Design review of the part built by this model. Coordinates are the model's own, in mm. A direction names the side the tool comes from. Give positions to 0.01 mm unless a question says otherwise; leave off trailing zeros. Write each loop counter-clockwise with the first axis right and the second up, starting at its lowest first coordinate (ties: lowest second). Pieces come first, ordered by that corner, then holes. Notation, with made-up numbers: M 70.25,52 L 87.25,52 A24 cw 87.25,63 Z; hole C -10.75,12 d4. An arc over 180 degrees is marked long. Answer in a Markdown table with one row per item.
Autodesk Inventor part; units mm, degrees
ref_plane "YZ Plane" through (0, 0, 0) normal (1, 0, 0) x (0, 1, 0)
ref_plane "XZ Plane" through (0, 0, 0) normal (0, 1, 0) x (-1, 0, 0)
ref_plane "XY Plane" through (0, 0, 0) normal (0, 0, 1) x (1, 0, 0)
sketch "Sketch1" plane through (0, 0, 0) normal (0, 0, 1) x (1, 0, 0)
  arc A0 (-25, 0) -> (25, 0) centre (0, 0) ccw
  circle A1 centre (0, 0) radius 2.5
  circle A2 centre (0, 15) radius 2.5
  line L0 (-25, 0) -> (-6, 0)
  line L1 (-6, 0) -> (-6, 15)
  arc A3 (6, 15) -> (-6, 15) centre (0, 15) ccw
  line L2 (6, 15) -> (6, 0)
  line L3 (6, 0) -> (25, 0)
  point P0 (0, 21)
  dimension "d0" = 50
  dimension "d1" = 5
  dimension "d2" = 15
  dimension "d4" = 12
extrude "Extrusion1" add sketch "Sketch1" along normal mid plane 8
hole "Hole1" at (0, 21, 0) direction (0, -1, 0) diameter 2.459 end up to surface
chamfer "Chamfer1" distance 0.5 angle 45 4 edges at (-2.5, 15, 4) (-2.5, 0, 4) (-2.5, 0, -4) (-2.5, 15, -4)
properties part number "Counterweight"
1) To check wall thickness, follow probe 1 along Y at (x, z) = (-1, 2.5); probe 2 along Z at (x, y) = (0, 19.2); probe 3 along X at (y, z) = (13, -1.25). State the ranges of each line that lie inside material, in increasing order. Write a range as [from, to].
Geometry says:
| item | result |
|---|---|
| probe 1 | [-24.98, -2.29], [2.29, 12.71], [17.29, 20.92] |
| probe 2 | [-4, -1.23], [1.23, 4] |
| probe 3 | [-6, -1.5], [1.5, 6] |
2) The part is to be moulded in two halves that separate along X. For faces 1 (the face through (6, 8, 0)), 2 (the face through (0.55, -24.994, -0.056)), 3 (the face through (15, 0, 0)), 4 (the face through (-0.54, 2.44, -0.05)), say which applies: released by +X, released by -X, zero draft, split by the parting line, or undercut.
Geometry says:
| item | result |
|---|---|
| face 1 | released by +X |
| face 2 | split by the parting line |
| face 3 | zero draft |
| face 4 | undercut |
3) For faces 5 (the face through (-16, 0, 0)), 6 (the face through (-1.22, 19.06, -0.16)), 7 (the face through (-0.33, 12.52, -0.05)), list the 3-axis set-ups (+Z, -Z, +X, -X, +Y, -Y) from which the entire face can be reached by the end or side of a thin tool; tool diameter is ignored.
Geometry says:
| item | result |
|---|---|
| face 5 | +Z, -Z, -X, +Y |
| face 6 | +Y |
| face 7 | +Z, -Z |
4) Add section B-B (z = 0.5). Write out the cut boundary in (x, y).
Geometry says:
| item | result |
|---|---|
| outline | M -25,0 A25 ccw 25,0 L 6,0 L 6,15 A6 ccw 1.12,20.89 L 1.12,17.23 A2.5 cw long -1.12,17.23 L -1.12,20.89 A6 ccw -6,15 L -6,0 Z; hole C 0,0 d5 |
5) Add section C-C (y = -9.5). Write out the cut boundary in (x, z), and give its area (3 significant figures).
Geometry says:
| item | result |
|---|---|
| outline | M -23.12,-4 L 23.12,-4 L 23.12,4 L -23.12,4 Z |
| area | 370 mm^2 |
6) Insertion check: P1, Ø1, axis at y = 4.5, z = 3, coming from the +X side; P2, Ø4.5, axis at x = 0, y = 15, coming from the -Z side; P3, Ø2.5, axis at x = -14.5, z = 1.5, coming from the +Y side; P4, Ø4, axis at y = -12, z = -2.5, coming from the -X side. Each pin has a flat end and moves straight along its axis. Give the tip position at first contact, or say it passes through.
Geometry says:
| item | result |
|---|---|
| P1 | x = 6 |
| P2 | through |
| P3 | y = 0 |
| P4 | x = -22.91 |
7) Add section A-A (x = 0). Write out the cut boundary in (y, z), and give its area (3 significant figures).
Geometry says:
| item | result |
|---|---|
| outline | M -25,-4 L -3,-4 L -2.5,-3.5 L -2.5,3.5 L -3,4 L -25,4 Z; M 2.5,-3.5 L 3,-4 L 12,-4 L 12.5,-3.5 L 12.5,3.5 L 12,4 L 3,4 L 2.5,3.5 Z; M 17.5,-3.5 L 18,-4 L 21,-4 L 21,-1.23 L 17.5,-1.23 Z; M 17.5,1.23 L 21,1.23 L 21,4 L 18,4 L 17.5,3.5 Z |
| area | 278 mm^2 |
8) Add section D-D (x = -21.5). Write out the cut boundary in (y, z).
Geometry says:
| item | result |
|---|---|
| outline | M -12.76,-4 L 0,-4 L 0,4 L -12.76,4 Z |
